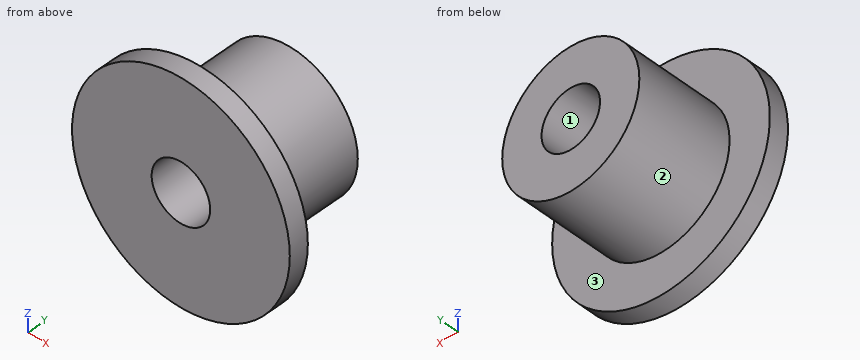
```python
from build123d import *

# Parameters (mm, degrees)
F0_R     = 89.2937
F1_DEPTH = 127
F2_R     = 141.749676
F3_DEPTH = 25.4
F5_D     = 76.2


with BuildPart() as f1:
    # F0 (on Front) → F1 (new body)
    with BuildSketch(Plane.XZ):
        Circle(F0_R)
    extrude(amount=F1_DEPTH)

    # F2 (on face) → F3 (join)
    with BuildSketch(Plane.XZ.offset(127)):
        Circle(F2_R)
    extrude(amount=F3_DEPTH)

    # F5 (through all)
    with Locations(Plane(origin=(0, 0, 0), x_dir=(-1, 0, 0), z_dir=(0, 1, 0))):
        with Locations((0, 0)):
            Hole(F5_D / 2)


solid = f1.part
```
The model under review builds one solid part; all positions refer to its coordinate system, in mm. Face numbers are marked on the shaded views. Round coordinates to 2 decimals unless told otherwise and drop trailing zeros. Write each loop counter-clockwise with the first axis right and the second up, starting at its lowest first coordinate (ties: lowest second). Pieces come first, ordered by that corner, then holes. Notation, with made-up numbers: M 88.25,-14.75 L 117.25,-14.75 A9 cw 117.25,1.25 Z; hole C -12.5,63 d6. An arc over 180 degrees is marked long. Use CSV: the item, a comma, the result in double quotes. Start each with the question number.
(1) We need section D-D, the plane x = -60.5. State the section outline as (y, z) points, then the cut area to 3 significant figures.
(2) For line 1 along Z through (x, y) = (-1, -90); line 2 along Y through (x, z) = (-113, 65.5); line 3 along X through (y, z) = (-27, -32), list the stretches that pass through material, from the lowest coordinate up.
(3) We need section B-B, the plane x = 0. State the section outline as (y, z) points.
(4) We need section C-C, the plane y = -137.5. State the section outline as (x, z) points.
(5) We need section A-A, the plane z = 0. State the section outline as (x, y) points, then the cut area to 3 significant figures.
(6) Clearance check with flat-ended pins moving along their axes: P1, Ø3, axis at y = -121.5, z = 68.5, coming from the +X side; P2, Ø1.5, axis at x = -63, y = -116.5, coming from the +Z side; P3, Ø5, axis at x = 36.5, y = -27, coming from the -Z side. State where each tip first meets the part, or that it passes through.
(7) The part is to be moulded in two halves that separate along Z. For the marked faces 1, 2 and 3, say which applies: +Z half, -Z half, draft (parallel to the pull), parting line (faces both ways), or undercut.
Findings:
1,outline,"M -152.4,-128.19 L -127,-128.19 L -127,-65.67 L 0,-65.67 L 0,65.67 L -127,65.67 L -127,128.19 L -152.4,128.19 Z"
1,area,"23,200 mm^2"
2,line 1,"-89.29 to -38.09, 38.09 to 89.29"
2,line 2,"-152.4 to -127"
2,line 3,"-83.36 to -20.68, 20.68 to 83.36"
3,outline,"M -152.4,-141.75 L -127,-141.75 L -127,-89.29 L 0,-89.29 L 0,-38.1 L -152.4,-38.1 Z; M -152.4,38.1 L 0,38.1 L 0,89.29 L -127,89.29 L -127,141.75 L -152.4,141.75 Z"
4,outline,"C 0,0 d283.5; hole C 0,0 d76.2"
5,outline,"M -141.75,-152.4 L -38.1,-152.4 L -38.1,0 L -89.29,0 L -89.29,-127 L -141.75,-127 Z; M 38.1,-152.4 L 141.75,-152.4 L 141.75,-127 L 89.29,-127 L 89.29,0 L 38.1,0 Z"
5,area,"18,300 mm^2"
6,P1,"x = 59.03"
6,P2,"z = 64.02"
6,P3,"z = -82.57"
7,face 1,"undercut"
7,face 2,"parting line"
7,face 3,"draft"
